Can you work these out from the model? Positions are in its coordinate system, mm. A direction names the side the tool comes from. Round coordinates to 2 decimals unless told otherwise and drop trailing zeros. Order: outer loops, then holes, each group sorted by start corner. A loop starts at its lowest first (then second) coordinate and runs counter-clockwise, first axis right, second up.
Q1. If I drill on line 1 (Y direction, x = -4, z = 10); line 2 (X direction, y = 55.5, z = -0.25), over which ranges is the centre line in solid material (lowest first)?
Q2. If we section it at D-D (z = 9.75): Please give me the cut outline in (x, y).
Q3. For faces 1 (the face through (0, 69.3, 0)), 2 (the face through (-0.2, 68.3, 7.5)), which set-ups out of +Z, -Z, +X, -X, +Y, -Y let a thin tool reach every point of the face, with its end or its side?
Q4. Will these pins go through, and if not, where does the flat tip stop? P1, Ø5, axis at y = 9.5, z = 2.5, coming from the -X side; P2, Ø5, axis at y = 26, z = -2.5, coming from the +X side; P3, Ø8, axis at x = 5, y = 17, coming from the +Z side.
Q5. If we section it at B-B (x = 0): Please give me the cut outline in (y, z), plus the area to 3 significant figures.
Q6. If we section it at A-A (z = 0): Please give me the cut outline in (x, y).
Q7. If we section it at C-C (y = 47.5): Please give me the cut outline in (x, z), plus the area to 3 significant figures.
Autodesk Inventor part; units mm, degrees
ref_plane "YZ Plane" through (0, 0, 0) normal (1, 0, 0) x (0, 1, 0)
ref_plane "XZ Plane" through (0, 0, 0) normal (0, 1, 0) x (-1, 0, 0)
ref_plane "XY Plane" through (0, 0, 0) normal (0, 0, 1) x (1, 0, 0)
sketch "Skizze1" plane through (0, 0, 0) normal (0, 0, 1) x (1, 0, 0)
  line L0 (0, 0) -> (5.15, 0)
  line L1 (5.15, 0) -> (5.15, 12)
  line L2 (0, 0) -> (0, 68.3)
  line L3 (0, 68.3) -> (7.15, 68.3)
  line L4 (7.15, 68.3) -> (7.15, 14)
  line L5 (5.15, 12) -> (5.15, 12)
  arc A0 (5.15, 12) -> (7.15, 14) centre (5.15, 14) ccw
  line L6 (7.15, 68.3) -> (11.4441, 68.3)
  line L7 (11.4441, 68.3) -> (11.4441, 69.3)
  line L8 (11.4441, 69.3) -> (0, 69.3)
  line L9 (0, 69.3) -> (0, 68.3)
  dimension "d0" = 5.15
  dimension "d1" = 12
  dimension "d2" = 68.3
  dimension "d3" = 7.15
  dimension "d4" = 2
  dimension "d5" = 1
revolve "Umdrehung1" add sketch "Skizze1" angle 360 about axis through (0, 0, 0) along (0, 1, 0)
properties part number "00_5ml_glue_cartridge"
Solution:
1. line 1: y = 68.3 to 69.3
1. line 2: x = -7.15 to 7.15
2. outline: (-5.99, 68.3) - (5.99, 68.3) - (5.99, 69.3) - (-5.99, 69.3) - close
3. face 1: +Z, -Z, +X, -X, +Y
3. face 2: -Y
4. P1: stops at x = -5.15
4. P2: stops at x = 7.15
4. P3: stops at z = 7.08
5. outline: (0, -5.15) - (12, -5.15) arc R2 ccw to (14, -7.15) - (68.3, -7.15) - (68.3, -11.44) - (69.3, -11.44) - (69.3, 11.44) - (68.3, 11.44) - (68.3, 7.15) - (14, 7.15) arc R2 ccw to (12, 5.15) - (0, 5.15) - close
5. area: 950 mm2
6. outline: (-11.44, 68.3) - (-7.15, 68.3) - (-7.15, 14) arc R2 ccw to (-5.15, 12) - (-5.15, 0) - (5.15, 0) - (5.15, 12) arc R2 ccw to (7.15, 14) - (7.15, 68.3) - (11.44, 68.3) - (11.44, 69.3) - (-11.44, 69.3) - close
7. outline: circle Ø14.3 at (0, 0)
7. area: 161 mm2
